Build history of the part. All positions in model axes, mm. A direction names the side the tool comes from. Give positions to 0.01 mm unless a question says otherwise; leave off trailing zeros. Order: outer loops, then holes, each group sorted by start corner. A loop starts at its lowest first (then second) coordinate and runs counter-clockwise, first axis right, second up. Notation, with made-up numbers: M 81,-8.5 L 127,-8.5 A13 cw 127,8.5 Z; hole C -31,38 d4. An arc over 180 degrees is marked long. One line per item, written item: value.
from build123d import *

# Parameters (mm, degrees)
SIDES_THE_GAP_VALUE_CAN_BE_CHANGED_DEPTH      = 228.6
BASE_DEPTH                                    = 3.175
SKETCH8_W                                     = 13.208
SKETCH8_H                                     = 1.524
SHOCK_CORD_CUTS_CAN_BE_MOVED_CURRENT_DI_DEPTH = 4.175


with BuildPart() as part:
    # Sketch3 → Sides (the gap value can be changed) (new body)
    with BuildSketch(Plane(origin=(0, 0, 0), x_dir=(1, 0, 0), z_dir=(0, 1, 0))):
        with BuildLine():
            ThreePointArc((-83.500112782, 12.664051105), (-84.455, 0), (-83.500112782, -12.664051105))
            ThreePointArc((-83.500112782, -12.664051105), (-36.842428798, -63.812958552), (30.782666419, -78.645244441))
            ThreePointArc((30.782666419, -78.645244441), (42.2275, -73.140175477), (52.717446363, -65.981193335))
            ThreePointArc((52.717446363, -65.981193335), (73.684857596, 0), (52.717446363, 65.981193335))
            ThreePointArc((52.717446363, 65.981193335), (42.2275, 73.140175477), (30.782666419, 78.645244441))
            ThreePointArc((30.782666419, 78.645244441), (-36.842428798, 63.812958552), (-83.500112782, 12.664051105))
        make_face()
        with BuildLine():
            ThreePointArc((50.384378709, 63.779720775), (70.509857596, 0), (50.384378709, -63.779720775))
            ThreePointArc((50.384378709, -63.779720775), (40.64, -70.39054482), (30.042669082, -75.524012303))
            ThreePointArc((30.042669082, -75.524012303), (-35.254928798, -61.063327895), (-80.427047792, -11.744291529))
            ThreePointArc((-80.427047792, -11.744291529), (-81.28, 0), (-80.427047792, 11.744291529))
            ThreePointArc((-80.427047792, 11.744291529), (-35.254928798, 61.063327895), (30.042669082, 75.524012303))
            ThreePointArc((30.042669082, 75.524012303), (40.64, 70.39054482), (50.384378709, 63.779720775))
        make_face(mode=Mode.SUBTRACT)
    extrude(amount=SIDES_THE_GAP_VALUE_CAN_BE_CHANGED_DEPTH)

    # Sketch7 → base (add)
    with BuildSketch(Plane(origin=(0, 0, 0), x_dir=(1, 0, 0), z_dir=(0, 1, 0))):
        with BuildLine():
            ThreePointArc((50.384378709, 63.779720775), (40.64, 70.39054482), (30.042669082, 75.524012303))
            ThreePointArc((30.042669082, 75.524012303), (-35.254928798, 61.063327895), (-80.427047792, 11.744291529))
            ThreePointArc((-80.427047792, 11.744291529), (-81.28, 0), (-80.427047792, -11.744291529))
            ThreePointArc((-80.427047792, -11.744291529), (-35.254928798, -61.063327895), (30.042669082, -75.524012303))
            ThreePointArc((30.042669082, -75.524012303), (40.64, -70.39054482), (50.384378709, -63.779720775))
            ThreePointArc((50.384378709, -63.779720775), (70.509857596, 0), (50.384378709, 63.779720775))
        make_face()
    extrude(amount=BASE_DEPTH)

    # Sketch8 → Shock cord cuts(Can be moved, current dim arbitrary) (cut, through all)
    with BuildSketch(Plane(origin=(0, 3.175, 0), x_dir=(1, 0, 0), z_dir=(0, 1, 0))):
        with Locations((0, 44.0055)):
            Rectangle(SKETCH8_W, SKETCH8_H)
        with Locations((0, -45.5295)):
            Rectangle(SKETCH8_W, SKETCH8_H)
    extrude(amount=-SHOCK_CORD_CUTS_CAN_BE_MOVED_CURRENT_DI_DEPTH, mode=Mode.SUBTRACT)


solid = part.part
1) Mould opens along X. For faces 1 (the face through (-81.28, 114.31, 0.16)), 2 (the face through (-34.429, 114.31, 61.535)), 3 (the face through (42.38, 112.7, -73.05)), 4 (the face through (-84.455, 112.7, -0.178)) say: released by +X, released by -X, zero draft, split by the parting line, or undercut.
Check values:
face 1: undercut
face 2: undercut
face 3: released by +X
face 4: released by -X
2) Saw through at C-C, the plane z = 7.5. Write the cut outline in (x, y) (3 decimals), then the cut area to 3 significant figures.
Check values:
outline: M -84.121,0 L 73.439,0 L 73.439,228.6 L 70.256,228.6 L 70.256,3.175 L -80.933,3.175 L -80.933,228.6 L -84.121,228.6 Z
area: 1,940 mm^2
3) Tool access for faces 5 (the face through (-36.08, 114.31, -60.58)), 6 (the face through (42.07, 112.7, 73.23)): list every direction of +Z, -Z, +X, -X, +Y, -Y with a clear straight run to the whole face (end or side of a thin tool).
Check values:
face 5: +Y
face 6: +Z, +X, +Y, -Y
4) Saw through at A-A, the plane y = 175.5. Write the cut outline in (x, z) (3 decimals).
Check values:
outline: M -83.5,-12.664 A114.3 ccw 30.783,-78.645 A84.455 ccw 52.717,-65.981 A114.3 ccw 52.717,65.981 A84.455 ccw 30.783,78.645 A114.3 ccw -83.5,12.664 A84.455 ccw Z; hole M -80.427,-11.744 A111.125 ccw 30.043,-75.524 A81.28 ccw 50.384,-63.78 A111.125 ccw 50.384,63.78 A81.28 ccw 30.043,75.524 A111.125 ccw -80.427,11.744 A81.28 ccw Z
5) Saw through at B-B, the plane x = -16. Write the cut outline in (y, z) (3 decimals), then the cut area to 3 significant figures.
Check values:
outline: M 0,-73.206 L 228.6,-73.206 L 228.6,-69.853 L 3.175,-69.853 L 3.175,69.853 L 228.6,69.853 L 228.6,73.206 L 0,73.206 Z
area: 1,980 mm^2
6) Pin check, flat tips, straight feed: pin 1 (10 mm diameter, centred on x = 14.5, y = 121, fed in from +Z); pin 2 (8 mm diameter, centred on x = 1, y = 171, fed in from -Z); pin 3 (6 mm diameter, centred on y = 69, z = -16, fed in from +X). Stop position of each tip, or through.
Check values:
pin 1: z = 79.12
pin 2: z = -78.1
pin 3: x = 72.94
7) Drill centre lines: probe 1 along Z at (x, y) = (10.5, 115.5); probe 2 along Z at (x, y) = (17, 191.5); probe 3 along Y at (x, z) = (33, -70) (3 decimals). Where is each one in solid material? Low to high. Write a range as from..to.
Check values:
probe 1: -78.7..-75.52, 75.52..78.7
probe 2: -79.08..-75.9, 75.9..79.08
probe 3: 0..3.175
